```python
from build123d import *

# Parameters (mm, degrees)
SKETCH2_W                  = 169.5
SKETCH2_H                  = 158
SKETCH2_R                  = 3
SKETCH2_W_2                = 26.88
SKETCH2_H_2                = 61.88
BOSS_EXTRUDE1_DEPTH        = 23
CUT_EXTRUDE1_DEPTH         = 189.415100244
CUT_EXTRUDE1_DEPTH_BACK    = 189.415100244
SKETCH3_W                  = 9.5
SKETCH3_H                  = 47
SKETCH4_R                  = 2
CUT_EXTRUDE2_DEPTH         = 7.5
SKETCH6_R                  = 14
CUT_EXTRUDE4_DEPTH         = 2
M10X1_0_TAPPED_HOLE1_D     = 9
M10X1_0_TAPPED_HOLE1_DEPTH = 10
M10X1_0_TAPPED_HOLE1_TIP   = 2.703872786


with BuildPart() as part:
    # Sketch2 → Boss-Extrude1 (new body)
    with BuildSketch(Plane.XY):
        with Locations((34.75, 0)):
            Rectangle(SKETCH2_W, SKETCH2_H)
        with Locations((29, -9)):
            Circle(SKETCH2_R, mode=Mode.SUBTRACT)
        with Locations((29, -24)):
            Circle(SKETCH2_R, mode=Mode.SUBTRACT)
        with BuildLine():
            Line((-5, 22), (-5, 5))
            ThreePointArc((-5, 5), (0, 0), (5, 5))
            Line((5, 5), (5, 22))
            ThreePointArc((5, 22), (0, 27), (-5, 22))
        make_face(mode=Mode.SUBTRACT)
        with Locations((58, 0)):
            Rectangle(SKETCH2_W_2, SKETCH2_H_2, mode=Mode.SUBTRACT)
    extrude(amount=BOSS_EXTRUDE1_DEPTH)

    # Sketch3 → Cut-Extrude1 (cut, two sides: drawn at the far end of the back side and taken through both)
    with BuildSketch(Plane(origin=(119.5, 0, 0), x_dir=(0, 0, -1), z_dir=(1, 0, 0)).offset(-CUT_EXTRUDE1_DEPTH_BACK)):
        with Locations((-4.75, 55.5)):
            Rectangle(SKETCH3_W, SKETCH3_H)
        with Locations((-4.75, -55.5)):
            Rectangle(SKETCH3_W, SKETCH3_H)
    extrude(amount=CUT_EXTRUDE1_DEPTH + CUT_EXTRUDE1_DEPTH_BACK, mode=Mode.SUBTRACT)

    # Sketch4 → Cut-Extrude2 (cut)
    with BuildSketch(Plane.XY):
        with Locations((74.5, -27)):
            Circle(SKETCH4_R)
        with Locations((74.5, 23)):
            Circle(SKETCH4_R)
        with Locations((27, 18.5)):
            Circle(SKETCH4_R)
        with Locations((27, 8.5)):
            Circle(SKETCH4_R)
    extrude(amount=CUT_EXTRUDE2_DEPTH, mode=Mode.SUBTRACT)

    # Sketch6 → Cut-Extrude4 (cut)
    with BuildSketch(Plane.XY.offset(23)):
        with Locations((103.5, 29)):
            Circle(SKETCH6_R)
        with Locations((103.5, -29)):
            Circle(SKETCH6_R)
        with Locations((-34, 29)):
            Circle(SKETCH6_R)
        with Locations((-34, -29)):
            Circle(SKETCH6_R)
    extrude(amount=-CUT_EXTRUDE4_DEPTH, mode=Mode.SUBTRACT)

    # M10x1.0 Tapped Hole1
    with Locations(Plane(origin=(0, 0, 21), x_dir=(0.9063077870366375, -0.42261826174072625, 0), z_dir=(0, 0, 1))):
        with Locations((-43.07039435, 11.913904925), (-18.558535169, -40.651946723), (81.546926368, 70.023915914), (106.058785549, 17.458064266)):
            Hole(M10X1_0_TAPPED_HOLE1_D / 2, depth=M10X1_0_TAPPED_HOLE1_DEPTH)
            with Locations((0, 0, -(M10X1_0_TAPPED_HOLE1_DEPTH + M10X1_0_TAPPED_HOLE1_TIP / 2))):  # 118° drill point
                Cone(0, M10X1_0_TAPPED_HOLE1_D / 2, M10X1_0_TAPPED_HOLE1_TIP, mode=Mode.SUBTRACT)


solid = part.part
```
For this review, take the finished solid that the model builds, in its own axes (mm). A direction names the side the tool comes from. Coordinates: 2 decimals unless noted, no trailing zeros. Write each loop counter-clockwise with the first axis right and the second up, starting at its lowest first coordinate (ties: lowest second). Pieces come first, ordered by that corner, then holes.
(1) For pin 1 Ø8 at (x, y) = (103.5, -29) entering from -Z; pin 2 Ø2.5 at (x, y) = (27, 18.5) entering from -Z; pin 3 Ø23.5 at (x, y) = (34, -53.5) entering from -Z; pin 4 Ø17 at (x, y) = (103.5, 29) entering from +Z, all flat-tipped, find the tip position at first contact; note any pin that passes through.
(2) Add section B-B on y = -9. Give the boundary of the cut face in (x, z), then the cut area to 3 significant figures.
(3) Add section C-C on z = 3. Count the separate pieces of the cut face and the enclosed holes in it, then the cut area to 3 significant figures.
(4) The part is to be moulded in two halves that separate along Y. For faces 1 (the face through (-50, -1, 14)), 2 (the face through (-34.763, -29.169, 8.766)), 3 (the face through (34, -79, 16)), say which applies: +Y half, -Y half, draft (parallel to the pull), parting line (faces both ways), or undercut.
(5) Tool access review of faces 4 (the face through (76.408, 23.601, 3.698)), 5 (the face through (0, 0, 11)), 6 (the face through (-37.3, -25.7, 21)): name each direction out of +Z, -Z, +X, -X, +Y, -Y from which nothing blocks a thin tool from reaching the whole face with its end or side.
(6) Add section D-D on x = 74.5. Give the boundary of the cut face in (y, z), then the cut area to 3 significant figures.
(7) Add section A-A on x = 0. Give the boundary of the cut face in (y, z).
(8) Wall thickness on probe 1 along Y at (x, z) = (74.5, 2.75); probe 2 along Y at (x, z) = (27, 3.75); probe 3 along Y at (x, z) = (103.5, 21.5): over which ranges is each line inside the solid? List them lowest first.
Answer sheet:
1. pin 1: stops at z = 0
1. pin 2: stops at z = 7.5
1. pin 3: stops at z = 9.5
1. pin 4: stops at z = 21
2. outline: (-50, 0) - (26, 0) - (26, 23) - (-50, 23) - close; (32, 0) - (44.56, 0) - (44.56, 23) - (32, 23) - close; (71.44, 0) - (119.5, 0) - (119.5, 23) - (71.44, 23) - close
2. area: 3,140 mm2
3. separate pieces: 1
3. enclosed holes: 8
3. area: 8,830 mm2
4. face 1: draft
4. face 2: undercut
4. face 3: -Y half
5. face 4: -Z
5. face 5: +Z, -Z
5. face 6: +Z
6. outline: (-79, 9.5) - (-32, 9.5) - (-32, 0) - (-29, 0) - (-29, 7.5) - (-25, 7.5) - (-25, 0) - (21, 0) - (21, 7.5) - (25, 7.5) - (25, 0) - (32, 0) - (32, 9.5) - (79, 9.5) - (79, 23) - (-79, 23) - close
6. area: 2,680 mm2
7. outline: (-79, 9.5) - (-32, 9.5) - (-32, 0) - (0, 0) - (0, 23) - (-79, 23) - close; (27, 0) - (32, 0) - (32, 9.5) - (79, 9.5) - (79, 23) - (27, 23) - close
8. probe 1: y = -32 to -29, -25 to 21, 25 to 32
8. probe 2: y = -32 to -26.24, -21.76 to -11.24, -6.76 to 6.5, 10.5 to 16.5, 20.5 to 32
8. probe 3: y = -79 to -43, -15 to 15, 43 to 79
